Read the model definition and answer for the solid it produces. Units are mm, in the model's axes. Face numbers are marked on the shaded views. Coordinates: 2 decimals unless noted, no trailing zeros. Order: outer loops, then holes, each group sorted by start corner. A loop starts at its lowest first (then second) coordinate and runs counter-clockwise, first axis right, second up.
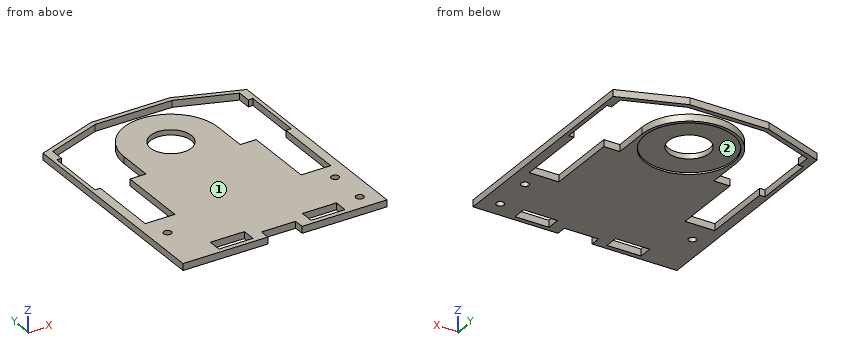
```python
from build123d import *

# Parameters (mm, degrees)
BOSS_EXTRUDE1_OUTLINE_W = 10
BOSS_EXTRUDE1_OUTLINE_H = 4
BOSS_EXTRUDE1_OUTLINE_R = 6
BOSS_EXTRUDE1_DEPTH     = 2
SKETCH2_R               = 12.875
CUT_EXTRUDE1_DEPTH      = 0.5
SKETCH3_R               = 1.125
CUT_EXTRUDE2_DEPTH      = 59.651581377
SKETCH4_W               = 10
SKETCH4_H               = 3
CUT_EXTRUDE3_DEPTH      = 59.651581377


# Read off the part's stored shape, not the designer's step: Boss-Extrude1
with BuildPart() as part:
    # Boss-Extrude1 outline → Boss-Extrude1 (new body)
    with BuildSketch(Plane.XY.offset(-369.35631811)):
        Polygon((-26.932250172, 41.859703988), (-26.932250172, -23.364250091), (32.867749828, -23.364250091), (32.867749828, 41.859703988), (14.52546441, 48.535749909), (-8.589964754, 48.535749909), align=None)
        with Locations((-10.532250172, -19.964250091)):
            Rectangle(BOSS_EXTRUDE1_OUTLINE_W, BOSS_EXTRUDE1_OUTLINE_H, mode=Mode.SUBTRACT)
        with Locations((16.467749828, -19.964250091)):
            Rectangle(BOSS_EXTRUDE1_OUTLINE_W, BOSS_EXTRUDE1_OUTLINE_H, mode=Mode.SUBTRACT)
        with BuildLine():
            Line((-25.782250172, 19.435749909), (-25.782250172, 37.235749909))
            Line((-25.782250172, 37.235749909), (-24.432250172, 37.235749909))
            Line((-24.432250172, 37.235749909), (-24.432250172, 41.279780692))
            Line((-24.432250172, 41.279780692), (-8.343106981, 47.135749909))
            Line((-8.343106981, 47.135749909), (14.278606637, 47.135749909))
            Line((14.278606637, 47.135749909), (30.367749828, 41.279780692))
            Line((30.367749828, 41.279780692), (30.367749828, 37.235749909))
            Line((30.367749828, 37.235749909), (31.717749828, 37.235749909))
            Line((31.717749828, 37.235749909), (31.717749828, 19.435749909))
            Line((31.717749828, 19.435749909), (30.167749828, 19.435749909))
            Line((30.167749828, 19.435749909), (30.167749828, -1.464250091))
            Line((30.167749828, -1.464250091), (21.467749828, -1.464250091))
            Line((21.467749828, -1.464250091), (21.467749828, 19.435749909))
            Line((21.467749828, 19.435749909), (16.767749828, 19.435749909))
            Line((16.767749828, 19.435749909), (16.767749828, 29.785749909))
            ThreePointArc((16.767749828, 29.785749909), (2.967749828, 43.585749909), (-10.832250172, 29.785749909))
            Line((-10.832250172, 29.785749909), (-10.832250172, 19.435749909))
            Line((-10.832250172, 19.435749909), (-15.532250172, 19.435749909))
            Line((-15.532250172, 19.435749909), (-15.532250172, -1.464250091))
            Line((-15.532250172, -1.464250091), (-24.232250172, -1.464250091))
            Line((-24.232250172, -1.464250091), (-24.232250172, 19.435749909))
            Line((-24.232250172, 19.435749909), (-25.782250172, 19.435749909))
        make_face(mode=Mode.SUBTRACT)
        with Locations((2.967749828, 29.785749909)):
            Circle(BOSS_EXTRUDE1_OUTLINE_R, mode=Mode.SUBTRACT)
    extrude(amount=BOSS_EXTRUDE1_DEPTH)

    # Sketch2 → Cut-Extrude1 (cut)
    with BuildSketch(Plane(origin=(0, 0, -369.35631811), x_dir=(-1, 0, 0), z_dir=(0, 0, -1))):
        with Locations((-2.967749828, 29.785749909)):
            Circle(SKETCH2_R)
    extrude(amount=-CUT_EXTRUDE1_DEPTH, mode=Mode.SUBTRACT)

    # Sketch3 → Cut-Extrude2 (cut, through all)
    with BuildSketch(Plane.XY.offset(-367.35631811)):
        with Locations((27.967749828, -6.964250091)):
            Circle(SKETCH3_R)
        with Locations((27.967749828, -18.464250091)):
            Circle(SKETCH3_R)
        with Locations((-21.932250172, -8.214250091)):
            Circle(SKETCH3_R)
    extrude(amount=-CUT_EXTRUDE2_DEPTH, mode=Mode.SUBTRACT)

    # Sketch4 → Cut-Extrude3 (cut, through all)
    with BuildSketch(Plane.XY.offset(-367.35631811)):
        with Locations((2.967749828, -21.864250091)):
            Rectangle(SKETCH4_W, SKETCH4_H)
    extrude(amount=-CUT_EXTRUDE3_DEPTH, mode=Mode.SUBTRACT)


solid = part.part
```
1) A cutting plane is placed at A-A, the plane y = 3.5. Determine the outline of the cut face in (x, z), and give its area (3 significant figures).
A:
outline: (-26.93, -369.36) - (-24.23, -369.36) - (-24.23, -367.36) - (-26.93, -367.36) - close; (-15.53, -369.36) - (21.47, -369.36) - (21.47, -367.36) - (-15.53, -367.36) - close; (30.17, -369.36) - (32.87, -369.36) - (32.87, -367.36) - (30.17, -367.36) - close
area: 84.8 mm2
2) Determine the mould class of the marked faces 1 and 2 for opening direction Y: pulls with the +Y half, pulls with the -Y half, needs draft (parallel to the pull), parting line crosses it, or undercut.
A:
face 1: needs draft
face 2: undercut
3) Straight lines are drawn through the part: line 1 (X direction, y = 16, z = -368.1); line 2 (X direction, y = 21, z = -368.55); line 3 (Y direction, x = 3, z = -367.95). For each, find the intervals that lie inside material, in ascending order.
A:
line 1: x = -26.93 to -24.23, -15.53 to 21.47, 30.17 to 32.87
line 2: x = -26.93 to -25.78, -10.83 to 16.77, 31.72 to 32.87
line 3: y = -20.36 to 23.79, 35.79 to 43.59, 47.14 to 48.54
4) Flat-ended cylindrical pins translate along their axes: pin 1 Ø0.6 at (x, z) = (-19, -368) entering from +Y; pin 2 Ø0.6 at (x, z) = (-13, -369) entering from +Y; pin 3 Ø0.5 at (x, z) = (31, -368.5) entering from +Y. Find the tip coordinate at first contact, or state that the pin passes through.
A:
pin 1: stops at y = 44.86
pin 2: stops at y = 47.04
pin 3: stops at y = 42.63
5) A cutting plane is placed at D-D, the plane z = -367.8. State how many separate pieces and enclosed holes the cut face has, and give its area (3 significant figures).
A:
separate pieces: 1
enclosed holes: 7
area: 2,690 mm2
6) A cutting plane is placed at C-C, the plane y = 38.5. Determine the outline of the cut face in (x, z), and give its area (3 significant figures).
A:
outline: (-26.93, -369.36) - (-24.43, -369.36) - (-24.43, -367.36) - (-26.93, -367.36) - close; (-7.73, -369.36) - (-6.51, -369.36) - (-6.51, -368.86) - (12.45, -368.86) - (12.45, -369.36) - (13.67, -369.36) - (13.67, -367.36) - (-7.73, -367.36) - close; (30.37, -369.36) - (32.87, -369.36) - (32.87, -367.36) - (30.37, -367.36) - close
area: 43.3 mm2
7) A cutting plane is placed at B-B, the plane x = 2. Determine the outline of the cut face in (y, z).
A:
outline: (-20.36, -369.36) - (16.95, -369.36) - (16.95, -368.86) - (23.86, -368.86) - (23.86, -367.36) - (-20.36, -367.36) - close; (35.71, -368.86) - (42.62, -368.86) - (42.62, -369.36) - (43.55, -369.36) - (43.55, -367.36) - (35.71, -367.36) - close; (47.14, -369.36) - (48.54, -369.36) - (48.54, -367.36) - (47.14, -367.36) - close
